```python
from build123d import *

# Parameters (mm, degrees)
BOSS_EXTRU_1_DEPTH      = 6
BOSS_EXTRU_2_DEPTH      = 12
ESQUISSE14_W            = 21
ESQUISSE14_H            = 6
ENL_V_MAT_EXTRU_2_DEPTH = 21
TROU_TARAUD_M81_D       = 6.8
TROU_TARAUD_M82_D       = 6.8
CONG_1_R                = 2


with BuildPart() as part:
    # Esquisse1 → Boss.-Extru.1 (new body)
    with BuildSketch(Plane(origin=(0, 0, 0), x_dir=(1, 0, 0), z_dir=(0, 1, 0))):
        with BuildLine():
            Line((0, 0), (0, 30))
            ThreePointArc((0, 30), (10, 40), (20, 30))
            Line((20, 30), (20, 0))
            ThreePointArc((20, 0), (10, -10), (0, 0))
        make_face()
    extrude(amount=BOSS_EXTRU_1_DEPTH)

    # Esquisse12 → Boss.-Extru.2 (add)
    with BuildSketch(Plane.XZ):
        with BuildLine():
            Line((0, -30), (20, -30))
            Line((20, -30), (20, 0))
            ThreePointArc((20, 0), (10, 10), (0, 0))
            Line((0, 0), (0, -30))
        make_face()
    extrude(amount=BOSS_EXTRU_2_DEPTH)

    # Esquisse14 → Enlèv. mat.-Extru.2 (cut, through all)
    with BuildSketch(Plane(origin=(20, 0, 0), x_dir=(0, 0, -1), z_dir=(1, 0, 0))):
        with Locations((0.5, 3)):
            Rectangle(ESQUISSE14_W, ESQUISSE14_H)
        Polygon((30, 0), (19, 0), (19, -6), (-10, -6), (-10, -12), (30, -12), align=None)
    extrude(amount=-ENL_V_MAT_EXTRU_2_DEPTH, mode=Mode.SUBTRACT)

    # Trou taraudé M81 (through all)
    with Locations(Plane(origin=(0, 6, 0), x_dir=(1, 0, 0), z_dir=(0, 1, 0))):
        with Locations((10, 30)):
            Hole(TROU_TARAUD_M81_D / 2)

    # Trou taraudé M82 (through all)
    with Locations(Plane(origin=(0, 0, 0), x_dir=(1, 0, 0), z_dir=(0, 1, 0))):
        with Locations((10, 0)):
            Hole(TROU_TARAUD_M82_D / 2)

    # Congé1
    cong_1_edges = [part.edges().sort_by_distance(p)[0] for p in [
        (10, -6, -19),
        (10, 6, -11),
    ]]
    fillet(cong_1_edges, radius=CONG_1_R)


solid = part.part
```
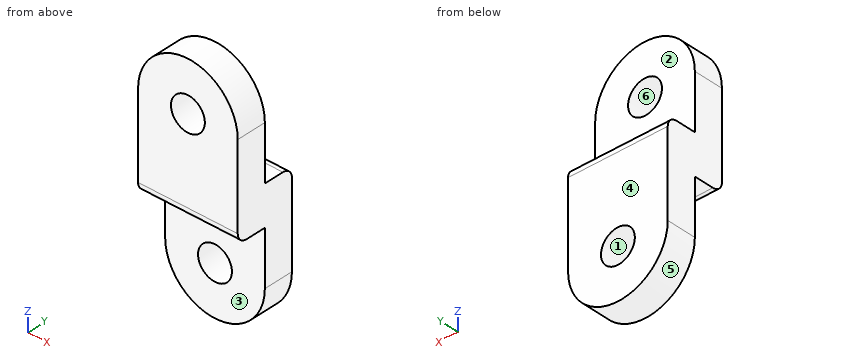
Can you work these out from the model? Positions are in its coordinate system, mm. Face numbers are marked on the shaded views. A direction names the side the tool comes from. Round coordinates to 2 decimals unless told otherwise and drop trailing zeros. Order: outer loops, then holes, each group sorted by start corner. A loop starts at its lowest first (then second) coordinate and runs counter-clockwise, first axis right, second up. Notation, with made-up numbers: (24.25, -1.75) -> (83.25, -1.75) arc R26 ccw to (83.25, 34.25) -> close; hole circle Ø9 at (21, 32). An arc over 180 degrees is marked (long way). Return JSON: item names as keys, results as strings. Group by question number.
1. I need wall thicknesses on line 1 (X direction, y = 1.35, z = -30); line 2 (Z direction, x = 10, y = 3.85); line 3 (Y direction, x = 3.25, z = -29.5). Which ranges of each line are inside material? Lowest first, please. Write a range as [from, to].
2. If we section it at A-A, the plane x = 10: Write out the boundary of the cut face in (y, z).
3. Will these pins go through, and if not, where does the flat tip stop? pin 1 (1.2 mm diameter, centred on x = 10, y = -1.5, fed in from -Z); pin 2 (5.5 mm diameter, centred on x = 10, z = 0, fed in from +Y); pin 3 (10 mm diameter, centred on x = 8, z = -26.5, fed in from -Y); pin 4 (4.5 mm diameter, centred on x = 11, y = 2.5, fed in from +Z).
4. If we section it at B-B, the plane z = 2: Write out the boundary of the cut face in (x, y), then the cut area to 3 significant figures.
5. If we section it at C-C, the plane y = 2.75: Write out the boundary of the cut face in (x, z).
6. We'd pull the mould along X, two halves only. Please class the marked faces 4, 5 and 6: released by +X, released by -X, zero draft, split by the parting line, or undercut.
7. Which directions (+Z, -Z, +X, -X, +Y, -Y) give clear straight access to the entire face, cutting with the end or side of a thin tool? Please do the marked faces 1, 2 and 3.
8. If we section it at D-D, the plane x = 5: Write out the boundary of the cut face in (y, z), then the cut area to 3 significant figures.
Output values:
{
 "1": {"line 1": "[0, 6.6], [13.4, 20]", "line 2": "[-40, -33.4], [-26.6, -11]", "line 3": "[0, 6]"},
 "2": {"outline": "(-6, -17) arc R2 ccw to (-4, -19) -> (0, -19) -> (0, -26.6) -> (6, -26.6) -> (6, -13) arc R2 ccw to (4, -11) -> (0, -11) -> (0, -3.4) -> (-6, -3.4) -> close; (-6, 3.4) -> (0, 3.4) -> (0, 10) -> (-6, 10) -> close; (0, -40) -> (6, -40) -> (6, -33.4) -> (0, -33.4) -> close"},
 "3": {"pin 1": "z = -19", "pin 2": "through", "pin 3": "y = 0", "pin 4": "z = -11"},
 "4": {"outline": "(0.2, -6) -> (7.25, -6) -> (7.25, 0) -> (0.2, 0) -> close; (12.75, -6) -> (19.8, -6) -> (19.8, 0) -> (12.75, 0) -> close", "area": "84.6 mm²"},
 "5": {"outline": "(0, -30) arc R10 ccw to (20, -30) -> (20, -11) -> (0, -11) -> close; hole circle Ø6.8 at (10, -30)"},
 "6": {"face 4": "zero draft", "face 5": "split by the parting line", "face 6": "undercut"},
 "7": {"face 1": "+Y, -Y", "face 2": "+Z, +X, -X, +Y", "face 3": "-Z, +X, -X, -Y"},
 "8": {"outline": "(-6, -17) arc R2 ccw to (-4, -19) -> (0, -19) -> (0, -38.66) -> (6, -38.66) -> (6, -13) arc R2 ccw to (4, -11) -> (0, -11) -> (0, 8.66) -> (-6, 8.66) -> close", "area": "330 mm²"}
}
